Could you check a few things on this model? Use its own coordinates, in mm. A direction names the side the tool comes from. Coordinates: 2 decimals unless noted, no trailing zeros. Write each loop counter-clockwise with the first axis right and the second up, starting at its lowest first coordinate (ties: lowest second). Pieces come first, ordered by that corner, then holes.
```python
from build123d import *

# Parameters (mm, degrees)
SZKIC1_W                                            = 90
SZKIC1_H                                            = 70
DODANIE_WYCI_GNI_CIE1_DEPTH                         = 6
SZKIC2_R                                            = 3
SZKIC2_R_2                                          = 0.95
DODANIE_WYCI_GNI_CIE2_DEPTH                         = 5
CBORE_FOR_M3_HEX_SOCKET_HEAD_CAP_SCREW1_D           = 3.2
CBORE_FOR_M3_HEX_SOCKET_HEAD_CAP_SCREW1_DEPTH       = 17.7
CBORE_FOR_M3_HEX_SOCKET_HEAD_CAP_SCREW1_CBORE_D     = 6.5
CBORE_FOR_M3_HEX_SOCKET_HEAD_CAP_SCREW1_CBORE_DEPTH = 3.4
CBORE_FOR_M3_HEX_SOCKET_HEAD_CAP_SCREW1_TIP         = 0.96137699


with BuildPart() as part:
    # Szkic1 → Dodanie-wyciągnięcie1 (new body)
    with BuildSketch(Plane(origin=(0, 0, 0), x_dir=(1, 0, 0), z_dir=(0, 1, 0))):
        Rectangle(SZKIC1_W, SZKIC1_H)
    extrude(amount=DODANIE_WYCI_GNI_CIE1_DEPTH)

    # Szkic2 → Dodanie-wyciągnięcie2 (add)
    # profile 1 of 4: a face of its own
    with BuildSketch(Plane(origin=(0, 6, 0), x_dir=(1, 0, 0), z_dir=(0, 1, 0))):
        with Locations(Location((-33, 23.2, 0), (0, 0, 270))):
            Circle(SZKIC2_R)
        with Locations(Location((-33, 23.2, 0), (0, 0, 270))):
            Circle(SZKIC2_R_2, mode=Mode.SUBTRACT)
    # profile 2 of 4: a face of its own
    with BuildSketch(Plane(origin=(0, 6, 0), x_dir=(1, 0, 0), z_dir=(0, 1, 0))):
        with Locations(Location((-33, -23.2, 0), (0, 0, 270))):
            Circle(SZKIC2_R)
        with Locations(Location((-33, -23.2, 0), (0, 0, 270))):
            Circle(SZKIC2_R_2, mode=Mode.SUBTRACT)
    # profile 3 of 4: a face of its own
    with BuildSketch(Plane(origin=(0, 6, 0), x_dir=(1, 0, 0), z_dir=(0, 1, 0))):
        with Locations(Location((33, -23.2, 0), (0, 0, 270))):
            Circle(SZKIC2_R)
        with Locations(Location((33, -23.2, 0), (0, 0, 270))):
            Circle(SZKIC2_R_2, mode=Mode.SUBTRACT)
    # profile 4 of 4: a face of its own
    with BuildSketch(Plane(origin=(0, 6, 0), x_dir=(1, 0, 0), z_dir=(0, 1, 0))):
        with Locations(Location((33, 23.2, 0), (0, 0, 270))):
            Circle(SZKIC2_R)
        with Locations(Location((33, 23.2, 0), (0, 0, 270))):
            Circle(SZKIC2_R_2, mode=Mode.SUBTRACT)
    extrude(amount=DODANIE_WYCI_GNI_CIE2_DEPTH)

    # CBORE for M3 Hex Socket Head Cap Screw1
    with Locations(Plane(origin=(0, 6, 0), x_dir=(1, 0, 0), z_dir=(0, 1, 0))):
        with Locations((-39, 29.1), (-39, -29.1), (39, 29.1), (39, -29.1)):
            CounterBoreHole(CBORE_FOR_M3_HEX_SOCKET_HEAD_CAP_SCREW1_D / 2, CBORE_FOR_M3_HEX_SOCKET_HEAD_CAP_SCREW1_CBORE_D / 2, CBORE_FOR_M3_HEX_SOCKET_HEAD_CAP_SCREW1_CBORE_DEPTH, depth=CBORE_FOR_M3_HEX_SOCKET_HEAD_CAP_SCREW1_DEPTH)
            with Locations((0, 0, -(CBORE_FOR_M3_HEX_SOCKET_HEAD_CAP_SCREW1_DEPTH + CBORE_FOR_M3_HEX_SOCKET_HEAD_CAP_SCREW1_TIP / 2))):  # 118° drill point
                Cone(0, CBORE_FOR_M3_HEX_SOCKET_HEAD_CAP_SCREW1_D / 2, CBORE_FOR_M3_HEX_SOCKET_HEAD_CAP_SCREW1_TIP, mode=Mode.SUBTRACT)


solid = part.part
```
1. If we mould it in two halves opening along Z, with no side actions, what happens to faces 3 (the face through (-1, 3, 35)), 4 (the face through (-33, 6, -23)), 5 (the face through (34, 11, 22))? For each: pulls with the +Z half, pulls with the -Z half, needs draft (parallel to the pull), parting line crosses it, or undercut.
Verdict:
face 3: pulls with the +Z half
face 4: undercut
face 5: needs draft
2. For pin 1 (5 mm diameter, centred on x = -33.5, z = 2, fed in from +Y); pin 2 (2.5 mm diameter, centred on x = -39, z = 29.1, fed in from -Y); pin 3 (3 mm diameter, centred on x = 37.5, z = 29.5, fed in from +Y), each with a flat end and sliding along its axis, tell me the tip position at first contact or that it passes through.
Verdict:
pin 1: stops at y = 6
pin 2: passes through
pin 3: stops at y = 2.6
3. Please list where these lines run through material, in increasing order: line 1 along Z through (x, y) = (39, 1.45); line 2 along X through (y, z) = (4.5, 29.1); line 3 along Z through (x, y) = (39, 5.2).
Verdict:
line 1: z = -35 to -30.7, -27.5 to 27.5, 30.7 to 35
line 2: x = -45 to -42.25, -35.75 to 35.75, 42.25 to 45
line 3: z = -35 to -32.35, -25.85 to 25.85, 32.35 to 35
4. I want a section at A-A on y = 8. Please give me the cut outline in (x, z), plus the area to 3 significant figures.
Verdict:
outline: circle Ø6 at (-33, -23.2); circle Ø6 at (-33, 23.2); circle Ø6 at (33, -23.2); circle Ø6 at (33, 23.2); hole circle Ø1.9 at (-33, -23.2); hole circle Ø1.9 at (-33, 23.2); hole circle Ø1.9 at (33, -23.2); hole circle Ø1.9 at (33, 23.2)
area: 102 mm2
5. On a 3-axis mill with a long thin cutter (end or side, diameter ignored), from which of +Z, -Z, +X, -X, +Y, -Y can I reach the whole of each face in a straight line? I mean faces 1 (the face through (-38, 2.6, -31)), 2 (the face through (-38.65, 1.28, 30.66)). Say none if no direction works.
Verdict:
face 1: +Y
face 2: +Y, -Y
6. I want a section at D-D on x = 33. Please give me the cut outline in (y, z).
Verdict:
outline: (0, -35) - (6, -35) - (6, -26.2) - (11, -26.2) - (11, -24.15) - (6, -24.15) - (6, -22.25) - (11, -22.25) - (11, -20.2) - (6, -20.2) - (6, 20.2) - (11, 20.2) - (11, 22.25) - (6, 22.25) - (6, 24.15) - (11, 24.15) - (11, 26.2) - (6, 26.2) - (6, 35) - (0, 35) - close
7. I want a section at C-C on z = -29.1. Please give me the cut outline in (x, y).
Verdict:
outline: (-45, 0) - (-40.6, 0) - (-40.6, 2.6) - (-42.25, 2.6) - (-42.25, 6) - (-45, 6) - close; (-37.4, 0) - (37.4, 0) - (37.4, 2.6) - (35.75, 2.6) - (35.75, 6) - (-35.75, 6) - (-35.75, 2.6) - (-37.4, 2.6) - close; (40.6, 0) - (45, 0) - (45, 6) - (42.25, 6) - (42.25, 2.6) - (40.6, 2.6) - close
8. I want a section at B-B on x = -39. Please give me the cut outline in (y, z).
Verdict:
outline: (0, -35) - (6, -35) - (6, -32.35) - (2.6, -32.35) - (2.6, -30.7) - (0, -30.7) - close; (0, -27.5) - (2.6, -27.5) - (2.6, -25.85) - (6, -25.85) - (6, 25.85) - (2.6, 25.85) - (2.6, 27.5) - (0, 27.5) - close; (0, 30.7) - (2.6, 30.7) - (2.6, 32.35) - (6, 32.35) - (6, 35) - (0, 35) - close
